Source: CAD feature listing. Evaluate the final solid. Frame: model axes, mm. A direction names the side the tool comes from. Coordinates: 2 decimals unless noted, no trailing zeros. Order: outer loops, then holes, each group sorted by start corner. A loop starts at its lowest first (then second) coordinate and runs counter-clockwise, first axis right, second up. Notation, with made-up numbers: (65.5, 89) -> (112.5, 89) arc R21 ccw to (112.5, 102) -> close; hole circle Ø8 at (-36, 27.25). An arc over 180 degrees is marked (long way). Write item = value, one per line. Start each with the question number.
Item 1: Set-up query: faces 1 (the flat face through (-10, 34, 2)), 2 (the flat face through (-10, 34, 0)). Return all of +Z, -Z, +X, -X, +Y, -Y with unobstructed straight access to the full face (end or side cutting, diameter ignored); none if empty.
Item 2: Contact query for flat-ended pins moving along their axis: pin 1 (0.6 mm diameter, centred on x = -500, z = 1.5, fed in from +Y); pin 2 (3 mm diameter, centred on x = -581.5, y = 9, fed in from +Z); pin 3 (3 mm diameter, centred on x = -562, z = 11.5, fed in from +Y); pin 4 (1.6 mm diameter, centred on x = 0.5, z = 1, fed in from +Y). Output: stop coordinate, or through.
Item 3: Ray query, line 1 along Z through (x, y) = (-230, 48); line 2 along Z through (x, y) = (-322, 3.5). Return the intervals inside material, ascending. Write a range as [from, to].
Item 4: Section query C-C (z = 12). Output: boundary loops of the cut face in (x, y).
Item 5: Section query A-A (y = 49.5). Output: boundary loops of the cut face in (x, z).
Item 6: Section query B-B (x = 250). Output: boundary loops of the cut face in (y, z).
Autodesk Inventor part; units mm, degrees
ref_plane "YZ Plane" through (0, 0, 0) normal (1, 0, 0) x (0, 1, 0)
ref_plane "XZ Plane" through (0, 0, 0) normal (0, 1, 0) x (-1, 0, 0)
ref_plane "XY Plane" through (0, 0, 0) normal (0, 0, 1) x (1, 0, 0)
sketch "Sketch1" plane through (0, 0, 0) normal (0, 0, 1) x (1, 0, 0)
  line L0 (-750, 62) -> (750, 62)
  line L1 (750, 62) -> (750, 0)
  line L2 (750, 0) -> (-750, 0)
  line L3 (-750, 0) -> (-750, 62)
  point P0 (0, 0)
  point P1 (0, 0)
  dimension "d0" = 1500
  dimension "d1" = 62
extrude "Plate1" add sketch "Sketch1" along normal blind 2
sketch "Sketch2" plane through (750, 2, 0) normal (0, -1, 0) x (1, 0, 0)
  line L0 (-1500, 0) -> (0, 0)
  line L1 (0, 0) -> (0, 20)
  line L2 (0, 20) -> (-1500, 20)
  line L3 (-1500, 20) -> (-1500, 0)
edge flange "Flange1" height 20 angle 90 thickness 2 bend radius 2.75 thickness toward (0, -1, 0) relief round relief width 2 relief depth 1 edges at (0, 0, 2) wall of the first edge with corners at (-750, 2, 0) (750, 2, 0) (750, 2, 20) (-750, 2, 20)
bend "Bend1"
corner "Corner1"
sketch "Sketch5" plane through (0, 0, 0) normal (0, 0, -1) x (-1, 0, 0)
  line L0 (750, 62) -> (-750, 62)
  line L1 (-1, 20) -> (-1, 62)
  line L2 (750, 0) -> (-750, 0)
  line L3 (-1, 20) -> (1, 20)
  line L4 (1, 20) -> (1, 62)
  point P0 (0, 0)
  point P1 (0, 20)
  point P2 (0, 0)
  dimension "d27" = 2
  dimension "d28" = 20
extrude "Extrusion1" cut sketch "Sketch5" against normal through all
pattern_linear "Rectangular Pattern1" count 3 spacing 500 along (1, 0, 0) of "Extrusion1" first direction both ways yes
sketch "Sketch6" plane through (0, 0, 0) normal (0, 0, -1) x (-1, 0, 0)
  line L0 (-750, 62) -> (-750, 4.75)
  circle A0 centre (-750, 62) radius 22.5
  line L1 (-750, 62) -> (750, 62)
  line L2 (-1, 20) -> (-1, 62)
  line L3 (-499, 62) -> (-499, 20)
  line L4 (-1, 20) -> (-499, 20) construction
  circle A1 centre (-250, 62) radius 22.5
  point P0 (0, 0)
  point P1 (-727.5, 62)
  point P2 (-750, 39.5)
  point P3 (-250, 20)
  dimension "d24" = 45
extrude "Extrusion2" cut sketch "Sketch6" along normal mid plane 30 contours L1 A0 L0 | A1 L1 | L1 A1 picked at (-748.3311, 47.188)
mirror "Mirror1" about plane through (0, 0, 0) normal (1, 0, 0) of "Extrusion2"
sketch "Sketch7" plane through (0, 0, 2) normal (0, 0, 1) x (1, 0, 0)
  arc A0 (-750, 39.5) -> (-727.5, 62) centre (-750, 62) ccw
  line L0 (-750, 4.75) -> (-750, 39.5)
  line L1 (-750, 4.75) -> (750, 4.75)
  line L2 (750, 39.5) -> (750, 4.75)
  arc A1 (727.5, 62) -> (750, 39.5) centre (750, 62) ccw
  line L3 (501, 62) -> (727.5, 62)
  line L4 (501, 62) -> (501, 20)
  line L5 (501, 20) -> (499, 20)
  line L6 (499, 20) -> (499, 62)
  line L7 (1, 62) -> (227.5, 62)
  line L8 (1, 62) -> (1, 20)
  line L9 (1, 20) -> (-1, 20)
  line L10 (-1, 20) -> (-1, 62)
  line L11 (-499, 62) -> (-272.5, 62)
  line L12 (-499, 62) -> (-499, 20)
  line L13 (-499, 20) -> (-501, 20)
  line L14 (-501, 20) -> (-501, 62)
  line L15 (-727.5, 62) -> (-501, 62)
  line L16 (650, 4.75) -> (650, 62) construction
  line L17 (-750, 4.75) -> (750, 4.75)
  circle A2 centre (650, 33.375) radius 5
  line L18 (272.5, 62) -> (499, 62)
  arc A3 (227.5, 62) -> (272.5, 62) centre (250, 62) ccw
  line L19 (-227.5, 62) -> (-1, 62)
  arc A4 (-272.5, 62) -> (-227.5, 62) centre (-250, 62) ccw
  point P0 (0, 0)
  dimension "d29" = 100
  dimension "d30" = 10
extrude "Extrusion3" [suppressed]
mirror "Mirror2" [suppressed]
sketch "Sketch8" plane through (0, 0, 2) normal (0, 0, 1) x (1, 0, 0)
  line L0 (494, 57) -> (494, 45) construction
  line L1 (494, 45) -> (294, 45) construction
  line L2 (294, 45) -> (294, 57) construction
  line L3 (294, 57) -> (494, 57) construction
  line L4 (501, 62) -> (727.5, 62)
  line L5 (272.5, 62) -> (499, 62)
  point P0 (0, 0)
  dimension "d33" = 200
  dimension "d34" = 12
  dimension "d37" = 5
  dimension "d38" = 5
mark "Mark2"
equation "\"d1\" = БОРТ_стрингер_3_высота"
equation "\"d27\" = d18"
equation "\"d2\" = Thickness"
equation "\"d3\" = BendReliefWidth"
equation "\"d4\" = BendReliefDepth"
equation "\"d5\" = MinimumRemnant"
equation "\"d6\" = TransitionRadius"
equation "\"d9\" = BendRadius"
equation "\"d10\" = CornerReliefSize"
equation "\"d11\" = GapSize"
equation "\"d12\" = JacobiRadiusSize"
equation "\"BendReliefWidth\" = Thickness"
equation "\"BendReliefDepth\" = 0.5 * Thickness"
equation "\"CornerReliefSize\" = 4 * Thickness"
equation "\"MinimumRemnant\" = 2 * Thickness"
equation "\"TransitionRadius\" = BendRadius"
equation "\"JacobiRadiusSize\" = BendRadius"
equation "\"GapSize\" = Thickness"
equation "\"d18\" = Thickness"
properties part number "MSC 316 stringer board #" material "Stainless Steel"
Computed:
q1.face_1 = +Z, +X, -X, +Y
q1.face_2 = -Z, +X, -X, +Y, -Y
q2.pin_1 = 20
q2.pin_2 = 2
q2.pin_3 = 2
q2.pin_4 = 62
q3.line_1 = [0, 2]
q3.line_2 = [0.17, 2.3]
q4.outline = (-750, 0) -> (750, 0) -> (750, 2) -> (-750, 2) -> close
q5.outline = (-731.29, 0) -> (-501, 0) -> (-501, 2) -> (-731.29, 2) -> close; (-499, 0) -> (-268.71, 0) -> (-268.71, 2) -> (-499, 2) -> close; (-231.29, 0) -> (-1, 0) -> (-1, 2) -> (-231.29, 2) -> close; (1, 0) -> (231.29, 0) -> (231.29, 2) -> (1, 2) -> close; (268.71, 0) -> (499, 0) -> (499, 2) -> (268.71, 2) -> close; (501, 0) -> (731.29, 0) -> (731.29, 2) -> (501, 2) -> close
q6.outline = (0, 4.75) arc R4.75 ccw to (4.75, 0) -> (39.5, 0) -> (39.5, 2) -> (4.75, 2) arc R2.75 cw to (2, 4.75) -> (2, 20) -> (0, 20) -> close
